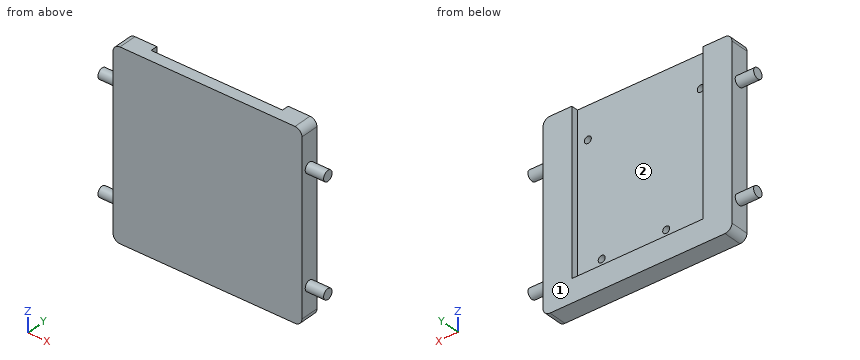
```python
from build123d import *

# Parameters (mm, degrees)
SKETCH1_W                = 82
SKETCH1_H                = 80
BOSS_EXTRUDE1_DEPTH      = 8
BOSS_EXTRUDE2_DEPTH      = 8
BOSS_EXTRUDE2_DEPTH_BACK = 90
SKETCH2_R                = 2.25
SKETCH3_W                = 57
SKETCH3_H                = 70
CUT_EXTRUDE1_DEPTH       = 3
SKETCH4_R                = 1.5
CUT_EXTRUDE2_DEPTH       = 3
FILLET1_R                = 3


with BuildPart() as part:
    # Sketch1 → Boss-Extrude1 (new body)
    with BuildSketch(Plane(origin=(0, 0, 0), x_dir=(1, 0, 0), z_dir=(0, 1, 0))):
        with Locations((0, 40)):
            Rectangle(SKETCH1_W, SKETCH1_H)
    extrude(amount=BOSS_EXTRUDE1_DEPTH)

    # Sketch2 → Boss-Extrude2 (add, two sides: drawn at the far end of the back side and taken through both)
    with BuildSketch(Plane(origin=(41, 0, 0), x_dir=(0, 0, -1), z_dir=(1, 0, 0)).offset(-BOSS_EXTRUDE2_DEPTH_BACK)):
        with Locations((17.5, 4)):
            Circle(SKETCH2_R)
        with Locations((65.5, 4)):
            Circle(SKETCH2_R)
    extrude(amount=BOSS_EXTRUDE2_DEPTH + BOSS_EXTRUDE2_DEPTH_BACK)

    # Sketch3 → Cut-Extrude1 (cut)
    with BuildSketch(Plane(origin=(0, 8, 0), x_dir=(1, 0, 0), z_dir=(0, 1, 0))):
        with Locations((0, 35)):
            Rectangle(SKETCH3_W, SKETCH3_H)
    extrude(amount=-CUT_EXTRUDE1_DEPTH, mode=Mode.SUBTRACT)

    # Sketch4 → Cut-Extrude2 (cut)
    with BuildSketch(Plane(origin=(0, 5, 0), x_dir=(1, 0, 0), z_dir=(0, 1, 0))):
        with Locations(Location((-25, 14, 0), (0, 0, 270))):
            Circle(SKETCH4_R)
        with Locations(Location((-10, 65, 0), (0, 0, 270))):
            Circle(SKETCH4_R)
        with Locations(Location((18, 65, 0), (0, 0, 270))):
            Circle(SKETCH4_R)
        with Locations(Location((24, 14, 0), (0, 0, 270))):
            Circle(SKETCH4_R)
    extrude(amount=-CUT_EXTRUDE2_DEPTH, mode=Mode.SUBTRACT)

    # Fillet1
    fillet1_edges = [part.edges().sort_by_distance(p)[0] for p in [
        (-41, 4, -80),
        (41, 4, -80),
        (41, 4, 0),
        (-41, 4, 0),
    ]]
    fillet(fillet1_edges, radius=FILLET1_R)


solid = part.part
```
Geometry: final body of the model. Coordinates: model frame, mm. Face numbers are marked on the shaded views. Give positions to 0.01 mm unless a question says otherwise; leave off trailing zeros. Write each loop counter-clockwise with the first axis right and the second up, starting at its lowest first coordinate (ties: lowest second). Pieces come first, ordered by that corner, then holes.
1. Section query C-C, the plane z = -65. Return loops of the section in (x, y).
2. Section query A-A, the plane x = 21. Return loops of the section in (y, z), then the cut area to 3 significant figures.
3. Section query B-B, the plane z = -7.5. Return loops of the section in (x, y).
4. Line query: probe 1 along X at (y, z) = (4.2, -14); probe 2 along X at (y, z) = (3.3, -65); probe 3 along X at (y, z) = (7, -55). Output: solid intervals per line, ascending.
5. Pin query (flat end, axial travel): P1, Ø3.5, axis at y = 6, z = -47.5, coming from the +X side; P2, Ø0.9, axis at x = -25.5, z = -13.5, coming from the +Y side; P3, Ø3.5, axis at x = 23.5, z = -14, coming from the +Y side. Return the tip coordinate at first contact, or that it passes through.
6. Draft query along X for the marked faces 1 and 2. Return one class per face: released by +X, released by -X, zero draft, split by the parting line, or undercut.
Computed:
1. outline: (-49, 1.81) - (-41, 1.81) - (-41, 0) - (41, 0) - (41, 1.81) - (49, 1.81) - (49, 6.19) - (41, 6.19) - (41, 8) - (28.5, 8) - (28.5, 5) - (19.5, 5) - (19.5, 2) - (16.5, 2) - (16.5, 5) - (-8.5, 5) - (-8.5, 2) - (-11.5, 2) - (-11.5, 5) - (-28.5, 5) - (-28.5, 8) - (-41, 8) - (-41, 6.19) - (-49, 6.19) - close
2. outline: (0, -80) - (8, -80) - (8, -70) - (5, -70) - (5, 0) - (0, 0) - close
2. area: 430 mm2
3. outline: (-41, 0) - (41, 0) - (41, 8) - (28.5, 8) - (28.5, 5) - (-28.5, 5) - (-28.5, 8) - (-41, 8) - close
4. probe 1: x = -41 to -26.5, -23.5 to 22.5, 25.5 to 41
4. probe 2: x = -49 to -11.5, -8.5 to 16.5, 19.5 to 49
4. probe 3: x = -41 to -28.5, 28.5 to 41
5. P1: stops at x = 41
5. P2: stops at y = 2
5. P3: stops at y = 5
6. face 1: zero draft
6. face 2: undercut
